The listing builds one solid part. Answer for the finished solid, in the listing's coordinates (mm). Face numbers are marked on the shaded views. A direction names the side the tool comes from. Round coordinates to 2 decimals unless told otherwise and drop trailing zeros. Write each loop counter-clockwise with the first axis right and the second up, starting at its lowest first coordinate (ties: lowest second). Pieces come first, ordered by that corner, then holes. Notation, with made-up numbers: M 62,-3 L 88,-3 A37 ccw 88,35 Z; hole C 54.5,84.25 d1. An arc over 180 degrees is marked long. Write each question's results on one line, items separated by ' | '.
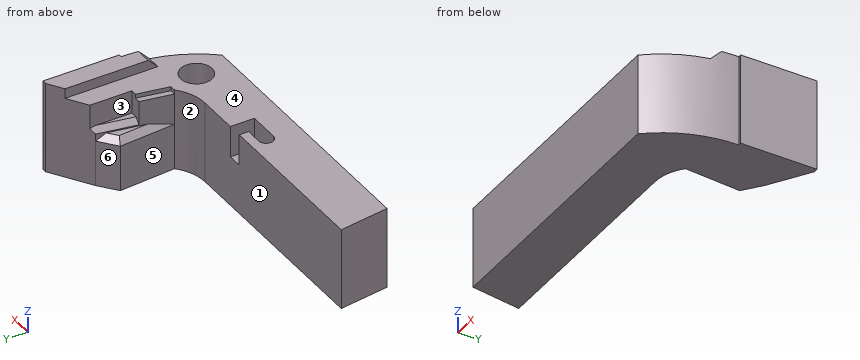
from build123d import *

# Parameters (mm, degrees)
F1_DEPTH  = 8.9
F2_W      = 28
F2_H      = 24.8338975774
F3_DEPTH  = 1.1
F4_W      = 81.2477835059
F4_H      = 5
F5_DEPTH  = 1.1
F6_R      = 1.5
F7_DEPTH  = 5.8
F8_W      = 8.6927097291
F8_H      = 13.0551015027
F9_DEPTH  = 0.15
F10_SIZE  = 0.9
F12_DEPTH = 3
F13_W     = 2.2015041194
F13_H     = 6.2
F14_DEPTH = 2.2
F15_SIZE  = 0.5
F17_DEPTH = 0.4
F19_DEPTH = 25
F21_DEPTH = 5
F22_SIZE  = 0.6


with BuildPart() as f1:
    # F0 (on Top) → F1 (new body)
    with BuildSketch(Plane.XY):
        with BuildLine():
            Line((-0.7, 4.8), (0, 0))
            Line((0, 0), (26, 0))
            ThreePointArc((26, 0), (28.1652277476, 3.687448042), (28.9, 7.9))
            Line((28.9, 7.9), (29.2, 7.9))
            Line((29.2, 7.9), (29.2, 15.2))
            Line((29.2, 15.2), (25.4, 15.2))
            Line((25.4, 15.2), (23.7, 5.9550013521))
            ThreePointArc((23.7, 5.9550013521), (22.3607712936, 5.0993739442), (20.8, 4.8))
            Line((20.8, 4.8), (-0.7, 4.8))
        make_face()
    extrude(amount=F1_DEPTH)

    # F2 (on face) → F3 (cut)
    with BuildSketch(Plane.XY.offset(8.9)):
        with Locations((13.3, 4.3441619959)):
            Rectangle(F2_W, F2_H)
    extrude(amount=-F3_DEPTH, mode=Mode.SUBTRACT)

    # F4 (on face) → F5 (cut)
    with BuildSketch(Plane.XY.offset(8.9)):
        with Locations((26.3764131814, 2.9)):
            Rectangle(F4_W, F4_H)
    extrude(amount=-F5_DEPTH, mode=Mode.SUBTRACT)

    # F6 (on face) → F7 (cut)
    with BuildSketch(Plane.XY.offset(7.8)):
        with Locations((24.8, 3.2)):
            Circle(F6_R)
    extrude(amount=-F7_DEPTH, mode=Mode.SUBTRACT)

    # F8 (on face) → F9 (cut)
    with BuildSketch(Plane.XY.offset(8.9)):
        with Locations((28.8734519854, 10.3571598884)):
            Rectangle(F8_W, F8_H)
    extrude(amount=-F9_DEPTH, mode=Mode.SUBTRACT)

    # F10
    f10_edges = [f1.edges().sort_by_distance(p)[0] for p in [
        (27.976572, 5.4, 8.75),
    ]]
    chamfer(f10_edges, length=F10_SIZE)

    # F11 (on face) → F12 (cut)
    with BuildSketch(Plane.XY.offset(7.8)):
        with BuildLine():
            ThreePointArc((13.8, 2.5), (14.2949747468, 2.7050252532), (14.5, 3.2))
            ThreePointArc((14.5, 3.2), (14.2949747468, 3.6949747468), (13.8, 3.9))
            ThreePointArc((13.8, 3.9), (13.1, 3.2), (13.8, 2.5))
        make_face()
        with BuildLine():
            ThreePointArc((13.8, 3.9), (14.2949747468, 3.6949747468), (14.5, 3.2))
            ThreePointArc((14.5, 3.2), (14.2949747468, 2.7050252532), (13.8, 2.5))
            Line((13.8, 2.5), (16.8, 2.5))
            Line((16.8, 2.5), (16.8, 4.8))
            Line((16.8, 4.8), (15.4, 4.8))
            Line((15.4, 4.8), (15.4, 3.9))
            Line((15.4, 3.9), (13.8, 3.9))
        make_face()
    extrude(amount=-F12_DEPTH, mode=Mode.SUBTRACT)

    # F13 (on face) → F14 (cut)
    with BuildSketch(Plane.XY.offset(7.8)):
        with Locations((24.2992479403, 12.1)):
            Rectangle(F13_W, F13_H)
    extrude(amount=-F14_DEPTH, mode=Mode.SUBTRACT)

    # F15
    f15_edges = [f1.edges().sort_by_distance(p)[0] for p in [
        (24.829962, 12.1, 5.6),
    ]]
    chamfer(f15_edges, length=F15_SIZE)

    # F16 (on face) → F17 (cut)
    with BuildSketch(Plane.XY.offset(7.8)):
        Polygon((24.8299620583, 9), (24.2599241167, 9), (23.7, 5.9550013521), (24.2599241167, 5.9550013521), align=None)
    extrude(amount=-F17_DEPTH, mode=Mode.SUBTRACT)

    # F18 (on face) → F19 (cut)
    with BuildSketch(Plane(origin=(0, 0, 0), x_dir=(1, 0, 0), z_dir=(0, 0, -1))):
        Polygon((28.7879798561, -15.2), (24.9478723404, -12.7412237639), (25.4, -15.2), align=None)
    extrude(amount=-F19_DEPTH, mode=Mode.SUBTRACT)

    # F20 (on face) → F21 (join)
    with BuildSketch(Plane(origin=(0, 0, 0), x_dir=(1, 0, 0), z_dir=(0, 0, -1))):
        Polygon((23.2760720335, -11.3907581303), (24.9478723404, -12.7412237639), (23.7, -5.9550013521), align=None)
    extrude(amount=-F21_DEPTH)

    # F22
    f22_edges = [f1.edges().sort_by_distance(p)[0] for p in [
        (23.488036, 8.67288, 5),
        (24.111972, 12.065991, 5),
    ]]
    chamfer(f22_edges, length=F22_SIZE)


solid = f1.part
1) Section D-D (x = 10.5) is taken. Determine the outline of the cut face in (y, z), then the cut area to 3 significant figures.
Return value:
outline: M 0,0 L 4.8,0 L 4.8,7.8 L 0,7.8 Z | area: 37.4 mm²
2) The mould has two halves that part along Y. Classify the marked faces 4, 5 and 6: +Y half, -Y half, draft (parallel to the pull), parting line (faces both ways), or undercut.
Return value:
face 4: draft | face 5: undercut | face 6: +Y half
3) Section C-C (y = 2) is taken. Determine the outline of the cut face in (x, z), then the cut area to 4 significant figures.
Return value:
outline: M -0.29,0 L 27.39,0 L 27.39,7.8 L 25.7,7.8 L 25.7,2 L 23.9,2 L 23.9,7.8 L -0.29,7.8 Z | area: 205.5 mm²
4) Section A-A (z = 1.5) is taken. Determine the outline of the cut face in (x, y) (3 decimals), then the cut area to 3 significant figures.
Return value:
outline: M -0.7,4.8 L 0,0 L 26,0 A12 ccw 28.9,7.9 L 29.2,7.9 L 29.2,15.2 L 28.788,15.2 L 24.948,12.741 L 23.276,11.391 L 23.7,5.955 A4.218 cw 20.8,4.8 Z | area: 183 mm²
5) Find the intervals of material crossed by line 1 (Y direction, x = 24.8, z = 6.3); line 2 (Z direction, x = 9.5, y = 2.75); line 3 (Y direction, x = 9.75, z = 1.75), in increasing order.
Return value:
line 1: 0 to 1.7, 4.7 to 9 | line 2: 0 to 7.8 | line 3: 0 to 4.8
6) Each of these flat-tipped pins is pushed along its axis until it touches: pin 1 (0.7 mm diameter, centred on x = 15, y = 3.5, fed in from +Z); pin 2 (1.2 mm diameter, centred on y = 12, z = 6.5, fed in from -X); pin 3 (0.7 mm diameter, centred on y = 4, z = 6.5, fed in from -X). Where does it stop, or does it pass through?
Return value:
pin 1: z = 4.8 | pin 2: x = 25.4 | pin 3: x = -0.63
7) A tool of negligible diameter and unlimited length cuts with its end or side. For the marked faces 1, 2 and 3, from which of +Z, -Z, +X, -X, +Y, -Y can it reach the whole face along a straight path? Write none if from no direction.
Return value:
face 1: +Z, -Z, -X, +Y | face 2: +Z, -Z, -X | face 3: +Z, -X, +Y
8) Section B-B (z = 2.75) is taken. Determine the outline of the cut face in (x, y) (3 decimals), then the cut area to 3 significant figures.
Return value:
outline: M -0.7,4.8 L 0,0 L 26,0 A12 ccw 28.9,7.9 L 29.2,7.9 L 29.2,15.2 L 28.788,15.2 L 24.948,12.741 L 23.276,11.391 L 23.7,5.955 A4.218 cw 20.8,4.8 Z; hole C 24.8,3.2 d3 | area: 176 mm²
